Autodesk Inventor part; units mm, degrees
ref_plane "YZ Plane" through (0, 0, 0) normal (1, 0, 0) x (0, 1, 0)
ref_plane "XZ Plane" through (0, 0, 0) normal (0, 1, 0) x (-1, 0, 0)
ref_plane "XY Plane" through (0, 0, 0) normal (0, 0, 1) x (1, 0, 0)
sketch "Skizze1" plane through (0, 0, 0) normal (0, 0, 1) x (1, 0, 0)
  circle A0 centre (0, 0) radius 32.5
  dimension "d0" = 65
extrude "Extrusion1" add sketch "Skizze1" along normal mid plane 25
sketch "Skizze2" plane through (0, 0, -12.5) normal (0, 0, -1) x (-1, 0, 0)
  circle A0 centre (0, 0) radius 25
  dimension "d3" = 50
extrude "Extrusion2" cut sketch "Skizze2" against normal blind 15
sketch "Skizze3" plane through (0, 0, 12.5) normal (0, 0, 1) x (1, 0, 0)
  point P0 (0, 0)
  point P1 (0, 0)
hole "Bohrung1" at (0, 0, 12.5) direction (0, 0, -1) diameter 4 end through all
properties part number "reifen"
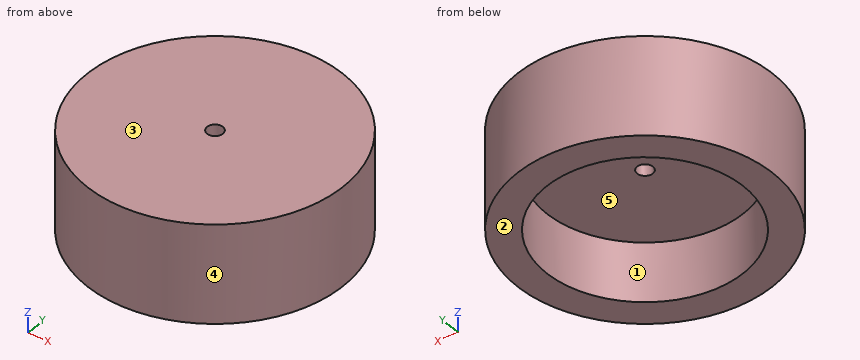
Source: CAD feature listing. Evaluate the final solid. Frame: model axes, mm. Face numbers are marked on the shaded views. A direction names the side the tool comes from. Round coordinates to 2 decimals unless told otherwise and drop trailing zeros. Loops run counter-clockwise (first coordinate to the right, second up) from the corner with the lowest first, then second, coordinate; pieces in that order, holes last. Notation, with made-up numbers: M 89.25,-16.75 L 122.25,-16.75 A18 ccw 122.25,2.25 Z; hole C -5.5,-5 d7. An arc over 180 degrees is marked long. Return JSON: item names as keys, results as strings. Group by question number.
1. Mould query, pull axis X, two halves, no side actions, for the marked faces 3, 4 and 5. Classes: released by +X, released by -X, zero draft, split by the parting line, or undercut.
2. Section query D-D on y = -19.5. Output: boundary loops of the cut face in (x, z).
3. Section query A-A on x = 0. Output: boundary loops of the cut face in (y, z), and give its area (3 significant figures).
4. Pin query (flat end, axial travel): pin 1 (4 mm diameter, centred on x = 0.5, y = -9.5, fed in from -Z); pin 2 (4 mm diameter, centred on y = -12, z = -3, fed in from -X); pin 3 (2 mm diameter, centred on x = -24, z = 8, fed in from -Y); pin 4 (3 mm diameter, centred on x = 0, y = 0, fed in from +Z). Return the tip coordinate at first contact, or that it passes through.
5. Section query C-C on z = 10.5. Output: boundary loops of the cut face in (x, y), and give its area (3 significant figures).
6. Reachability of the marked faces 1 and 2 from +Z, -Z, +X, -X, +Y, -Y: full face, straight path, thin tool, end or side. Return the list, or none.
7. Material intervals for line 1 along Y through (x, z) = (0, -7.25); line 2 along Y through (x, z) = (0, 8.75); line 3 along X through (y, z) = (10, 0), sorted ascending. Write a range as from..to.
Checks:
{
 "1": {"face 3": "zero draft", "face 4": "split by the parting line", "face 5": "undercut"},
 "2": {"outline": "M -26,-12.5 L -15.64,-12.5 L -15.64,2.5 L 15.64,2.5 L 15.64,-12.5 L 26,-12.5 L 26,12.5 L -26,12.5 Z"},
 "3": {"outline": "M -32.5,-12.5 L -25,-12.5 L -25,2.5 L -2,2.5 L -2,12.5 L -32.5,12.5 Z; M 2,2.5 L 25,2.5 L 25,-12.5 L 32.5,-12.5 L 32.5,12.5 L 2,12.5 Z", "area": "835 mm²"},
 "4": {"pin 1": "stops at z = 2.5", "pin 2": "stops at x = -30.92", "pin 3": "stops at y = -22.96", "pin 4": "passes through"},
 "5": {"outline": "C 0,0 d65; hole C 0,0 d4", "area": "3,310 mm²"},
 "6": {"face 1": "-Z", "face 2": "-Z, +X, -X, +Y, -Y"},
 "7": {"line 1": "y = -32.5..-25, 25..32.5", "line 2": "y = -32.5..-2, 2..32.5", "line 3": "x = -30.92..-22.91, 22.91..30.92"}
}
